```python
from build123d import *

# Parameters (mm, degrees)
F6_DEPTH  = 19.05
F1_R      = 15.875
F0_R      = 41.275
F8_R      = 34.925
F9_DEPTH  = 31.75
F10_R     = 25.4
F11_DEPTH = 12.7
F12_R     = 9.525
F13_DEPTH = 50.8
F15_DEPTH = 12.7
F16_R     = 9.525
F17_DEPTH = 25.4


with BuildPart() as f6:
    # F2 (on Top) → F6 (new body)
    with BuildSketch(Plane.XY):
        Polygon((-20.5864672744, 35.7746137668), (-60.1274476785, 12.8457909373), (-27.6046618819, 7.8555336222), align=None)
    extrude(amount=F6_DEPTH)


with BuildPart() as f6b:
    # F1 (on Top) → F6, piece 2 (new body)
    with BuildSketch(Plane.XY):
        with Locations((-50.8, 0)):
            Circle(F1_R)
    extrude(amount=F6_DEPTH)


with BuildPart() as f6c:
    # F1 (on Top) → F6, piece 3 (new body)
    with BuildSketch(Plane.XY):
        with Locations((50.8, 0)):
            Circle(F1_R)
    extrude(amount=F6_DEPTH)


with BuildPart() as f6d:
    # F0 (on Top) → F6, piece 4 (new body)
    with BuildSketch(Plane.XY):
        Circle(F0_R)
    extrude(amount=F6_DEPTH)


with BuildPart() as f6e:
    # F3 (on Top) → F6, piece 5 (new body)
    with BuildSketch(Plane.XY):
        Polygon((-30.2489809692, -6.1483276077), (-60.227651149, -12.5827733427), (-21.6209739447, -35.1033322513), align=None)
    extrude(amount=F6_DEPTH)


with BuildPart() as f6f:
    # F4 (on Top) → F6, piece 6 (new body)
    with BuildSketch(Plane.XY):
        Polygon((58.4153184481, 13.6340273871), (17.3395914771, 37.4561636104), (25.2016615123, 3.7444084883), align=None)
    extrude(amount=F6_DEPTH)


with BuildPart() as f6g:
    # F5 (on Top) → F6, piece 7 (new body)
    with BuildSketch(Plane.XY):
        Polygon((28.4536294639, -4.6330923215), (20.3704475493, -35.8993813455), (59.0077042557, -13.5921507853), align=None)
    extrude(amount=F6_DEPTH)


with BuildPart() as f6_1:
    add(f6.part)

    # F7: union F6d, F6e, F6g, F6f, F6c, F6b
    add(f6d.part)
    add(f6e.part)
    add(f6g.part)
    add(f6f.part)
    add(f6c.part)
    add(f6b.part)

    # F8 (on face) → F9 (join)
    with BuildSketch(Plane.XY.offset(19.05)):
        Circle(F8_R)
    extrude(amount=F9_DEPTH)

    # F10 (on face) → F11 (cut)
    with BuildSketch(Plane.XY.offset(50.8)):
        Circle(F10_R)
    extrude(amount=-F11_DEPTH, mode=Mode.SUBTRACT)

    # F12 (on face) → F13 (cut)
    with BuildSketch(Plane.XY.offset(38.1)):
        Circle(F12_R)
    extrude(amount=-F13_DEPTH, mode=Mode.SUBTRACT)

    # F14 (on face) → F15 (cut)
    with BuildSketch(Plane.XY.offset(50.8)):
        with BuildLine():
            Line((-34.3428758988, -6.35), (-24.5934442484, -6.35))
            ThreePointArc((-24.5934442484, -6.35), (-25.4, 0), (-24.5934442484, 6.35))
            Line((-24.5934442484, 6.35), (-34.3428758988, 6.35))
            ThreePointArc((-34.3428758988, 6.35), (-34.925, 0), (-34.3428758988, -6.35))
        make_face()
        with BuildLine():
            Line((-6.35, 34.3428758988), (-6.35, 24.5934442484))
            ThreePointArc((-6.35, 24.5934442484), (0, 25.4), (6.35, 24.5934442484))
            Line((6.35, 24.5934442484), (6.35, 34.3428758988))
            ThreePointArc((6.35, 34.3428758988), (0, 34.925), (-6.35, 34.3428758988))
        make_face()
        with BuildLine():
            ThreePointArc((25.4, 0), (25.1975542852, -3.2005090291), (24.5934442484, -6.35))
            Line((24.5934442484, -6.35), (34.3428758988, -6.35))
            ThreePointArc((34.3428758988, -6.35), (34.7791644937, -3.1883133656), (34.925, 0))
            ThreePointArc((34.925, 0), (34.7791644937, 3.1883133656), (34.3428758988, 6.35))
            Line((34.3428758988, 6.35), (24.5934442484, 6.35))
            ThreePointArc((24.5934442484, 6.35), (25.1975542852, 3.2005090291), (25.4, 0))
        make_face()
        with BuildLine():
            ThreePointArc((6.35, -24.5934442484), (0, -25.4), (-6.35, -24.5934442484))
            Line((-6.35, -24.5934442484), (-6.35, -34.3428758988))
            ThreePointArc((-6.35, -34.3428758988), (0, -34.925), (6.35, -34.3428758988))
            Line((6.35, -34.3428758988), (6.35, -24.5934442484))
        make_face()
    extrude(amount=-F15_DEPTH, mode=Mode.SUBTRACT)

    # F16 (on face) → F17 (cut)
    with BuildSketch(Plane.XY.offset(19.05)):
        with Locations((-50.8, 0)):
            Circle(F16_R)
        with Locations((50.8, 0)):
            Circle(F16_R)
    extrude(amount=-F17_DEPTH, mode=Mode.SUBTRACT)


solid = f6_1.part
```
Model file for the job. Use its own axes, mm. A direction names the side the tool comes from. Coordinates: 2 decimals unless noted, no trailing zeros. Order: outer loops, then holes, each group sorted by start corner. A loop starts at its lowest first (then second) coordinate and runs counter-clockwise, first axis right, second up. Notation, with made-up numbers: (-1.5, 42) -> (10.5, 42) arc R15 ccw to (10.5, 50) -> close; hole circle Ø8 at (34, -26.5). An arc over 180 degrees is marked (long way). Return JSON: item names as keys, results as strings.
Item 1: Slice it at A-A (x = 0). Write the cut outline in (y, z) (3 decimals).
Model answer:
{"outline": "(-41.275, 0) -> (-9.525, 0) -> (-9.525, 38.1) -> (-34.925, 38.1) -> (-34.925, 19.05) -> (-41.275, 19.05) -> close; (9.525, 0) -> (41.275, 0) -> (41.275, 19.05) -> (34.925, 19.05) -> (34.925, 38.1) -> (9.525, 38.1) -> close"}
Item 2: Slice it at C-C (z = 7.5). Count the separate pieces of the cut face and the enclosed holes in it, then the cut area to 3 significant figures.
Model answer:
{"separate pieces": "1", "enclosed holes": "3", "area": "6,470 mm²"}
Item 3: Pin check, flat tips, straight feed: P1, Ø5, axis at y = 5, z = 39, coming from the -X side; P2, Ø3, axis at x = 28.5, z = 43, coming from the -Y side; P3, Ø10.5, axis at x = 29.5, z = 46, coming from the +Y side. Stop position of each tip, or through.
Model answer:
{"P1": "stops at x = -34.82", "P2": "stops at y = -22.15", "P3": "stops at y = 25.13"}
Item 4: 3-axis set-ups, long thin cutter, end or side, ignore diameter. For faces 4 (the face through (6.35, -30, 45)), 5 (the face through (7, 8, 38.1)), 6 (the face through (30, 6.35, 45)), 7 (the face through (20, 21, 50.8)), 8 (the face through (40.25, 24.17, 9.39)): which of +Z, -Z, +X, -X, +Y, -Y reach the whole face in a straight line?
Model answer:
{"face 4": "+Z, +Y, -Y", "face 5": "+Z", "face 6": "+Z, +X, -X", "face 7": "+Z, +X, -X, +Y, -Y", "face 8": "+Z, -Z, +X, +Y"}
Item 5: Slice it at B-B (y = 0). Write the cut outline in (x, z) (3 decimals), then the cut area to 3 significant figures.
Model answer:
{"outline": "(-66.675, 0) -> (-60.325, 0) -> (-60.325, 19.05) -> (-66.675, 19.05) -> close; (-41.275, 0) -> (-9.525, 0) -> (-9.525, 38.1) -> (-34.925, 38.1) -> (-34.925, 19.05) -> (-41.275, 19.05) -> close; (9.525, 0) -> (41.275, 0) -> (41.275, 19.05) -> (34.925, 19.05) -> (34.925, 38.1) -> (9.525, 38.1) -> close; (60.325, 0) -> (66.675, 0) -> (66.675, 19.05) -> (60.325, 19.05) -> close", "area": "2,420 mm²"}
Item 6: Mould opens along X. For faces 1 (the face through (-39.68, -24.57, 9.39)), 2 (the face through (-30, -6.35, 45)), 3 (the face through (-6.35, 30, 45)) say: pulls with the +X half, pulls with the -X half, needs draft (parallel to the pull), parting line crosses it, or undercut.
Model answer:
{"face 1": "pulls with the -X half", "face 2": "needs draft", "face 3": "undercut"}
Item 7: Wall check: line 1 along Y through (x, z) = (0, 18) (3 decimals); line 2 along Z through (x, y) = (-4, 19); line 3 along Z through (x, y) = (43.5, -8.5). Give the ranges that are in metal, low to high. Write a range as from..to.
Model answer:
{"line 1": "y = -41.275..-9.525, 9.525..41.275", "line 2": "z = 0..38.1", "line 3": "z = 0..19.05"}
Item 8: Slice it at D-D (x = 50.8). Write the cut outline in (y, z) (3 decimals), then the cut area to 3 significant figures.
Model answer:
{"outline": "(-18.331, 0) -> (-9.525, 0) -> (-9.525, 19.05) -> (-18.331, 19.05) -> close; (9.525, 0) -> (18.051, 0) -> (18.051, 19.05) -> (9.525, 19.05) -> close", "area": "330 mm²"}
